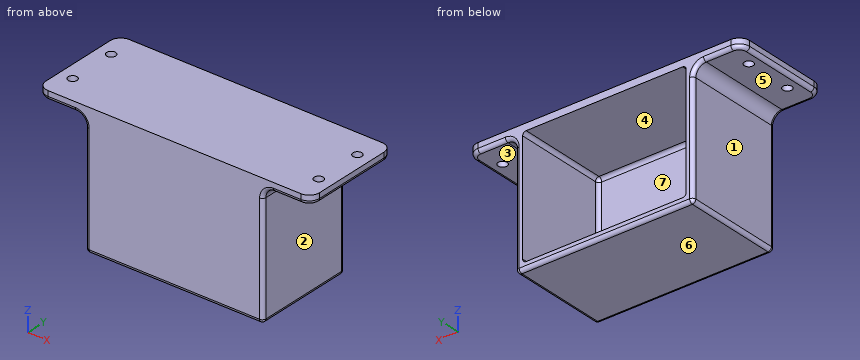
```python
from build123d import *

# Parameters (mm, degrees)
SKETCH1_W           = 129.54
SKETCH1_H           = 96.52
BOSS_EXTRUDE1_DEPTH = 73.66
SKETCH2_W           = 119.38
SKETCH2_H           = 86.36
CUT_EXTRUDE1_DEPTH  = 68.58
FILLET1_R           = 2.54
SKETCH3_W           = 35.179
SKETCH3_H           = 73.66
SKETCH3_R           = 3.302
BOSS_EXTRUDE2_DEPTH = 6.35
FILLET2_R           = 7.62
FILLET3_R           = 7.62
FILLET4_R           = 7.62
FILLET5_R           = 2.54


with BuildPart() as part:
    # Sketch1 → Boss-Extrude1 (new body)
    with BuildSketch(Plane(origin=(0, 0, 0), x_dir=(1, 0, 0), z_dir=(0, 1, 0))):
        Rectangle(SKETCH1_W, SKETCH1_H)
    extrude(amount=BOSS_EXTRUDE1_DEPTH)

    # Sketch2 → Cut-Extrude1 (cut)
    with BuildSketch(Plane(origin=(0, 73.66, 0), x_dir=(1, 0, 0), z_dir=(0, 1, 0))):
        Rectangle(SKETCH2_W, SKETCH2_H)
    extrude(amount=-CUT_EXTRUDE1_DEPTH, mode=Mode.SUBTRACT)

    # Fillet1
    fillet1_edges = [part.edges().sort_by_distance(p)[0] for p in [
        (59.69, 5.08, 0),
        (59.69, 39.37, -43.18),
        (0, 5.08, 43.18),
        (59.69, 39.37, 43.18),
        (-59.69, 5.08, 0),
        (-59.69, 39.37, 43.18),
        (0, 5.08, -43.18),
        (-59.69, 39.37, -43.18),
    ]]
    fillet(fillet1_edges, radius=FILLET1_R)

    # Sketch3 → Boss-Extrude2 (add)
    # profile 1 of 2: a face of its own
    with BuildSketch(Plane.XY.offset(48.26)):
        with Locations((-82.3595, 36.83)):
            Rectangle(SKETCH3_W, SKETCH3_H)
        with Locations((-89.916, 54.356)):
            Circle(SKETCH3_R, mode=Mode.SUBTRACT)
        with Locations(Location((-89.916, 19.304, 0), (0, 0, 180))):
            Circle(SKETCH3_R, mode=Mode.SUBTRACT)
    # profile 2 of 2: a face of its own
    with BuildSketch(Plane.XY.offset(48.26)):
        with Locations((82.3595, 36.83)):
            Rectangle(SKETCH3_W, SKETCH3_H)
        with Locations((89.916, 19.304)):
            Circle(SKETCH3_R, mode=Mode.SUBTRACT)
        with Locations(Location((89.916, 54.356, 0), (0, 0, 180))):
            Circle(SKETCH3_R, mode=Mode.SUBTRACT)
    extrude(amount=-BOSS_EXTRUDE2_DEPTH)

    # Fillet2
    fillet2_edges = [part.edges().sort_by_distance(p)[0] for p in [
        (-64.77, 36.83, 41.91),
        (64.77, 36.83, 41.91),
    ]]
    fillet(fillet2_edges, radius=FILLET2_R)

    # Fillet3
    fillet3_edges = [part.edges().sort_by_distance(p)[0] for p in [
        (-99.949, 73.66, 45.085),
        (-99.949, 0, 45.085),
    ]]
    fillet(fillet3_edges, radius=FILLET3_R)

    # Fillet4
    fillet4_edges = [part.edges().sort_by_distance(p)[0] for p in [
        (99.949, 73.66, 45.085),
        (99.949, 0, 45.085),
    ]]
    fillet(fillet4_edges, radius=FILLET4_R)

    # Fillet5
    fillet5_edges = [part.edges().sort_by_distance(p)[0] for p in [
        (-64.77, 73.66, -6.985),
        (-99.949, 36.83, 41.91),
        (-82.3595, 0, 41.91),
        (-97.717153673, 2.231846327, 41.91),
        (-97.717153673, 71.428153673, 41.91),
        (99.949, 36.83, 41.91),
        (82.3595, 73.66, 41.91),
        (97.717153673, 2.231846327, 41.91),
        (97.717153673, 71.428153673, 41.91),
        (-64.77, 0, -6.985),
        (0, 0, -48.26),
        (0, 73.66, -48.26),
        (-64.77, 36.83, -48.26),
        (64.77, 36.83, -48.26),
        (64.77, 73.66, -6.985),
        (64.77, 0, -6.985),
        (82.3595, 0, 41.91),
        (-82.3595, 73.66, 41.91),
        (67.001846327, 0, 39.678153673),
        (67.001846327, 73.66, 39.678153673),
        (-67.001846327, 73.66, 39.678153673),
        (-67.001846327, 0, 39.678153673),
    ]]
    fillet(fillet5_edges, radius=FILLET5_R)


solid = part.part
```
Geometry check sheet. Reference: the model listing, model coordinates, mm. Face numbers are marked on the shaded views. A direction names the side the tool comes from. Coordinates: 2 decimals unless noted, no trailing zeros. Loops run counter-clockwise (first coordinate to the right, second up) from the corner with the lowest first, then second, coordinate; pieces in that order, holes last. Notation, with made-up numbers: (83, 82) - (91, 82) arc R14 ccw to (91, 98) - close; hole circle Ø4 at (85.25, 69). An arc over 180 degrees is marked (long way). One line per item, written item: value. Start each with the question number.
(1) Cross-section at A-A on y = 39. Enter the section's corners in (x, z), plus the area to 3 significant figures.
(2) Depth check by flat-ended pin: P1, Ø1.5, axis at y = 58, z = 20.5, coming from the +X side; P2, Ø3, axis at x = -18, z = -15, coming from the +Y side; P3, Ø12.5, axis at x = 81, y = 52.5, coming from the -Z side. Enter the tip coordinate at first touch or a pass-through.
(3) Tool access check on the marked faces 5, 6 and 7. Record the directions out of +Z, -Z, +X, -X, +Y, -Y that give a thin tool (end or side, any length) a straight path to the whole face; none if there is none.
(4) Cross-section at C-C on x = -29.5. Enter the section's corners in (y, z), plus the area to 3 significant figures.
(5) Material ranges on line 1 (X direction, y = 52, z = 28); line 2 (Z direction, x = 18, y = 36); line 3 (Y direction, x = 37.5, z = -25), recorded low to high. Write a range as [from, to].
(6) Cross-section at B-B on z = -31.5. Enter the section's corners in (x, y), plus the area to 3 significant figures.
(7) Mould release check, pull along X, two halves, no side actions. Record for the marked faces 1, 2, 3 and 4: released by +X, released by -X, zero draft, split by the parting line, or undercut.
Results below:
1. outline: (-99.95, 44.45) arc R2.54 ccw to (-97.41, 41.91) - (-72.39, 41.91) arc R7.62 cw to (-64.77, 34.29) - (-64.77, -45.72) arc R2.54 ccw to (-62.23, -48.26) - (62.23, -48.26) arc R2.54 ccw to (64.77, -45.72) - (64.77, 34.29) arc R7.62 cw to (72.39, 41.91) - (97.41, 41.91) arc R2.54 ccw to (99.95, 44.45) - (99.95, 48.26) - (-99.95, 48.26) - close; hole (-59.69, -40.64) arc R2.54 ccw to (-57.15, -43.18) - (57.15, -43.18) arc R2.54 ccw to (59.69, -40.64) - (59.69, 40.64) arc R2.54 ccw to (57.15, 43.18) - (-57.15, 43.18) arc R2.54 ccw to (-59.69, 40.64) - close
1. area: 2,670 mm2
2. P1: stops at x = 64.77
2. P2: stops at y = 5.08
2. P3: stops at z = 41.91
3. face 5: -Z, -X, +Y, -Y
3. face 6: -Z, +X, -X, +Y, -Y
3. face 7: +Y
4. outline: (0, -45.72) arc R2.54 ccw to (2.54, -48.26) - (71.12, -48.26) arc R2.54 ccw to (73.66, -45.72) - (73.66, -43.18) - (7.62, -43.18) arc R2.54 cw to (5.08, -40.64) - (5.08, 40.64) arc R2.54 cw to (7.62, 43.18) - (73.66, 43.18) - (73.66, 48.26) - (0, 48.26) - close
4. area: 1,190 mm2
5. line 1: x = [-64.77, -59.69], [59.69, 64.77]
5. line 2: z = [-48.26, -43.18], [43.18, 48.26]
5. line 3: y = [0, 5.08]
6. outline: (-64.77, 2.54) arc R2.54 ccw to (-62.23, 0) - (62.23, 0) arc R2.54 ccw to (64.77, 2.54) - (64.77, 71.12) arc R2.54 ccw to (62.23, 73.66) - (59.69, 73.66) - (59.69, 7.62) arc R2.54 cw to (57.15, 5.08) - (-57.15, 5.08) arc R2.54 cw to (-59.69, 7.62) - (-59.69, 73.66) - (-62.23, 73.66) arc R2.54 ccw to (-64.77, 71.12) - close
6. area: 1,350 mm2
7. face 1: released by -X
7. face 2: released by +X
7. face 3: zero draft
7. face 4: undercut
